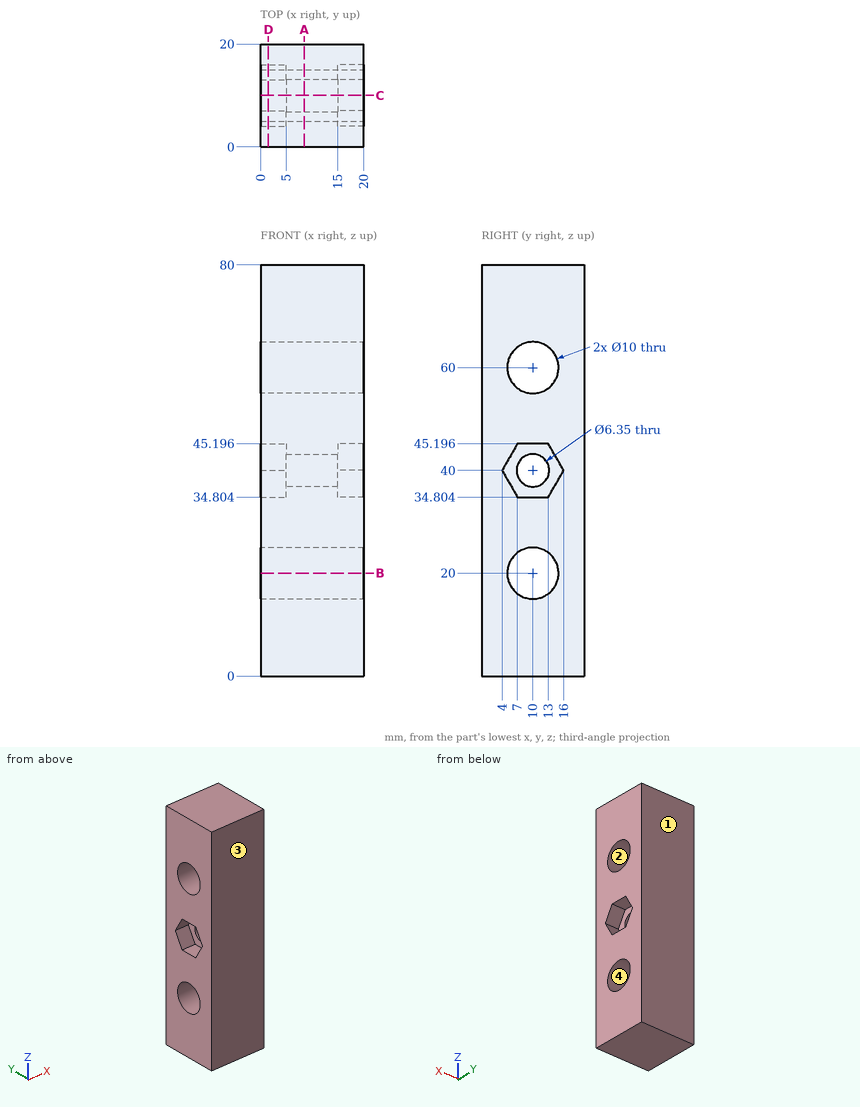
The figure shows three views and two pictorial views of one solid part (mm, origin at its lowest corner). Answer the questions. Round coordinates to 2 decimals unless told otherwise and drop trailing zeros. Order: outer loops, then holes, each group sorted by start corner. A loop starts at its lowest first (then second) coordinate and runs counter-clockwise, first axis right, second up. Notation, with made-up numbers: M 26,-14 L 32,-14 A20 cw 32,13 Z; hole C 77.5,-18 d7. An arc over 180 degrees is marked long. Put each result on its own line as item: value. Start each with the question number.
Q1. A flat-ended cylindrical pin translates along its axis: pin 1 (5 mm diameter, centred on y = 10, z = 37.5, fed in from +X). Find the tip coordinate at first contact, or state that the pin passes through.
Q2. Section D-D, the plane x = 1.5 is taken. Write down the section's boundary in (y, z), and give its area (3 significant figures).
Q3. Section A-A, the plane x = 8.5 is taken. Write down the section's boundary in (y, z) (3 decimals).
Q4. Straight lines are drawn through the part: L1, parallel to Y at x = 10.25, z = 40 (3 decimals); L2, parallel to Z at x = 13, y = 6; L3, parallel to Z at x = 12.75, y = 6.5. For each, find the intervals that lie inside material, in ascending order. Write a range as [from, to].
Q5. For a pull along Y with two mould halves and no side action, classify the marked faces 1, 2, 3 and 4 as pulls with the +Y half, pulls with the -Y half, needs draft (parallel to the pull), parting line crosses it, or undercut.
Q6. Section C-C, the plane y = 10 is taken. Write down the section's boundary in (x, z) (3 decimals).
Q7. Section B-B, the plane z = 20 is taken. Write down the section's boundary in (x, y), and give its area (3 significant figures).
Findings below:
1. pin 1: stops at x = 15
2. outline: M 0,0 L 20,0 L 20,80 L 0,80 Z; hole M 4,40 L 7,34.8 L 13,34.8 L 16,40 L 13,45.2 L 7,45.2 Z; hole C 10,20 d10; hole C 10,60 d10
2. area: 1,350 mm^2
3. outline: M 0,0 L 20,0 L 20,80 L 0,80 Z; hole C 10,20 d10; hole C 10,60 d10; hole C 10,40 d6.35
4. L1: y = [0, 6.825], [13.175, 20]
4. L2: z = [0, 17], [23, 57], [63, 80]
4. L3: z = [0, 16.43], [23.57, 56.43], [63.57, 80]
5. face 1: pulls with the +Y half
5. face 2: undercut
5. face 3: pulls with the -Y half
5. face 4: undercut
6. outline: M 0,0 L 20,0 L 20,15 L 0,15 Z; M 0,25 L 20,25 L 20,34.804 L 15,34.804 L 15,36.825 L 5,36.825 L 5,34.804 L 0,34.804 Z; M 0,45.196 L 5,45.196 L 5,43.175 L 15,43.175 L 15,45.196 L 20,45.196 L 20,55 L 0,55 Z; M 0,65 L 20,65 L 20,80 L 0,80 Z
7. outline: M 0,0 L 20,0 L 20,5 L 0,5 Z; M 0,15 L 20,15 L 20,20 L 0,20 Z
7. area: 200 mm^2
